Autodesk Inventor part; units mm, degrees
ref_plane "YZ Plane" through (0, 0, 0) normal (1, 0, 0) x (0, 1, 0)
ref_plane "XZ Plane" through (0, 0, 0) normal (0, 1, 0) x (-1, 0, 0)
ref_plane "XY Plane" through (0, 0, 0) normal (0, 0, 1) x (1, 0, 0)
sketch "スケッチ1" plane through (0, 0, 0) normal (0, 0, 1) x (1, 0, 0)
  line L0 (-4, 17.75) -> (4, 17.75)
  line L1 (4, 17.75) -> (4, -17.75)
  line L2 (4, -17.75) -> (-4, -17.75)
  line L3 (-4, -17.75) -> (-4, 17.75)
  line L4 (-4, 17.75) -> (4, -17.75) construction
  line L5 (4, 17.75) -> (-4, -17.75) construction
  point P0 (0, 0)
  dimension "d0" = 8
  dimension "d1" = 35.5
extrude "押し出し1" add sketch "スケッチ1" along normal blind 0.55
sketch "スケッチ2" plane through (0, 0, 0.55) normal (0, 0, 1) x (1, 0, 0)
  line L0 (-4, -17.75) -> (4, -17.75)
  line L1 (3, -17.75) -> (3, 2.75)
  line L2 (4, -17.75) -> (4, 17.75)
  line L3 (3, -17.75) -> (23.5, -17.75) construction
  line L4 (0, -17.75) -> (-3, -17.75)
  line L5 (-3, -17.75) -> (-3, 2.75)
  line L6 (-4, 17.75) -> (-4, -17.75)
  line L7 (-4, 4.25) -> (-3, 2.75)
  line L8 (-4, 4.25) -> (-4, -17.75)
  line L9 (-4, -17.75) -> (-3, -17.75)
  line L10 (4, 4.25) -> (3, 2.75)
  line L11 (4, 4.25) -> (4, -17.75)
  line L12 (3, -17.75) -> (4, -17.75)
  point P0 (0, 0)
  dimension "d4" = 20.5
  dimension "d5" = 90
  dimension "d6" = 3
extrude "押し出し2" cut sketch "スケッチ2" against normal blind 0.55
sketch "スケッチ3" plane through (0, 0, 0.55) normal (0, 0, 1) x (1, 0, 0)
  circle A0 centre (0, -12.5) radius 1.25
  circle A1 centre (0, -10) radius 1.25
  line L0 (1.25, -10) -> (1.25, -12.5)
  line L1 (-1.25, -10) -> (-1.25, -12.5)
  point P0 (0, 0)
  dimension "d9" = 2.5
extrude "押し出し3" cut sketch "スケッチ3" against normal blind 10
sketch "スケッチ4" plane through (-4, 17.75, 0) normal (-1, 0, 0) x (0, 0, 1)
  line L0 (0.55, 0) -> (0.55, -13.5)
  line L1 (0.55, 0) -> (0.55, -1.5)
  line L2 (0, -13.5) -> (0, 0)
  line L3 (0.55, -1.5) -> (0, 0)
  line L4 (0, 0) -> (0.55, 0)
  point P0 (0, -17.75)
  dimension "d12" = 1.5
extrude "押し出し4" cut sketch "スケッチ4" against normal blind 10
properties part number "pen_type_cutter_realsize" material "鋼、合金鋼"
Read the model definition and answer for the solid it produces. Units are mm, in the model's axes. A direction names the side the tool comes from. Give positions to 0.01 mm unless a question says otherwise; leave off trailing zeros. Write each loop counter-clockwise with the first axis right and the second up, starting at its lowest first coordinate (ties: lowest second). Pieces come first, ordered by that corner, then holes. Notation, with made-up numbers: (66, -30) - (91, -30) arc R28 cw to (91, -7) - close; hole circle Ø3 at (-15, 70.5). An arc over 180 degrees is marked (long way). Return JSON: item names as keys, results as strings.
Q1. For faces 1 (the face through (-0.03, -13.75, 0.28)), 2 (the face through (-3.5, 3.5, 0.3)), determine the directions among +Z, -Z, +X, -X, +Y, -Y from which every point of the face is accessible in a straight line to the end or side of a thin tool.
Reply:
{"face 1": "+Z, -Z", "face 2": "+Z, -Z, -X, -Y"}
Q2. A cutting plane is placed at C-C, the plane y = 1.5. Determine the outline of the cut face in (x, z), and give its area (3 significant figures).
Reply:
{"outline": "(-3, 0) - (3, 0) - (3, 0.55) - (-3, 0.55) - close", "area": "3.30 mm²"}
Q3. A cutting plane is placed at D-D, the plane x = -2.5. Determine the outline of the cut face in (y, z), and give its area (3 significant figures).
Reply:
{"outline": "(-17.75, 0) - (17.75, 0) - (16.25, 0.55) - (-17.75, 0.55) - close", "area": "19.1 mm²"}
Q4. Consider line 1 along X through (y, z) = (2, 0.2); line 2 along X through (y, z) = (-11.5, 0.5); line 3 along X through (y, z) = (-13.5, 0.2). Determine where each line is inside the solid, lowest interval first. Write a range as [from, to].
Reply:
{"line 1": "[-3, 3]", "line 2": "[-3, -1.25], [1.25, 3]", "line 3": "[-3, -0.75], [0.75, 3]"}
Q5. A cutting plane is placed at B-B, the plane z = 0.2. Determine the outline of the cut face in (x, y), and give its area (3 significant figures).
Reply:
{"outline": "(-4, 4.25) - (-3, 2.75) - (-3, -17.75) - (3, -17.75) - (3, 2.75) - (4, 4.25) - (4, 17.2) - (-4, 17.2) - close; hole (-1.25, -12.5) arc R1.25 ccw to (1.25, -12.5) - (1.25, -10) arc R1.25 ccw to (-1.25, -10) - close", "area": "226 mm²"}
Q6. A cutting plane is placed at A-A, the plane x = 0. Determine the outline of the cut face in (y, z), and give its area (3 significant figures).
Reply:
{"outline": "(-17.75, 0) - (-13.75, 0) - (-13.75, 0.55) - (-17.75, 0.55) - close; (-8.75, 0) - (17.75, 0) - (16.25, 0.55) - (-8.75, 0.55) - close", "area": "16.4 mm²"}
Q7. For a pull along X with two mould halves and no side action, classify faces 3 (the face through (0.03, -8.75, 0.28)), 4 (the face through (3.5, 3.5, 0.3)), 5 (the face through (0, 0, 0)) as released by +X, released by -X, zero draft, split by the parting line, or undercut.
Reply:
{"face 3": "undercut", "face 4": "released by +X", "face 5": "zero draft"}
